Autodesk Inventor part; units mm, degrees
ref_plane "YZ Plane" through (0, 0, 0) normal (1, 0, 0) x (0, 1, 0)
ref_plane "XZ Plane" through (0, 0, 0) normal (0, 1, 0) x (-1, 0, 0)
ref_plane "XY Plane" through (0, 0, 0) normal (0, 0, 1) x (1, 0, 0)
sketch "Sketch1" plane through (0, 0, 0) normal (0, 1, 0) x (-1, 0, 0)
  line L0 (51, -51) -> (-51, -51)
  line L1 (-51, -51) -> (-51, 51)
  line L2 (-51, 51) -> (51, 51)
  line L3 (51, 51) -> (51, -51)
  line L4 (51, -51) -> (-51, 51) construction
  line L5 (-51, -51) -> (51, 51) construction
  point P0 (0, 0)
  dimension "d0" = 102
  dimension "d1" = 102
extrude "Extrusion1" add sketch "Sketch1" along normal blind 17
chamfer "Chamfer1" distance 15 angle 45 4 edges at (51, 8.5, 51) (51, 8.5, -51) (-51, 8.5, -51) (-51, 8.5, 51)
sketch "Sketch2" plane through (0, 17, 0) normal (0, 1, 0) x (1, 0, 0)
  line L0 (51, -36) -> (51, 36)
  line L1 (-51, 36) -> (-51, -36)
  line L2 (51, -36) -> (36, -51)
  line L3 (36, 51) -> (-36, 51)
  circle A0 centre (36, -36) radius 6.5
  circle A1 centre (-36, -36) radius 6.5
  circle A2 centre (36, 36) radius 6.5
  circle A3 centre (-36, 36) radius 6.5
  circle A4 centre (0, 0) radius 23
  dimension "d7" = 13
  dimension "d8" = 13
  dimension "d9" = 13
  dimension "d10" = 13
  dimension "d22" = 46
extrude "Extrusion2" cut sketch "Sketch2" against normal through all contours A0 | A1 | A2 | A3
thread "Thread1"
thread "Thread2"
thread "Thread3"
thread "Thread4"
sketch "Sketch3" plane through (0, 17, 0) normal (0, 1, 0) x (1, 0, 0)
  circle A0 centre (0, 0) radius 23
  dimension "d23" = 46
extrude "Extrusion3" cut sketch "Sketch3" against normal through all
properties part number "00.32.004 \"Flange\"" material "Steel"
Read the model definition and answer for the solid it produces. Units are mm, in the model's axes. Coordinates: 2 decimals unless noted, no trailing zeros. Loops run counter-clockwise (first coordinate to the right, second up) from the corner with the lowest first, then second, coordinate; pieces in that order, holes last.
(1) The part is cut by section B-B (y = 5.75). Determine the outline of the cut face in (x, z), and give its area (3 significant figures).
Solution:
outline: (-51, -36) - (-36, -51) - (36, -51) - (51, -36) - (51, 36) - (36, 51) - (-36, 51) - (-51, 36) - close; hole circle Ø13 at (-36, -36); hole circle Ø13 at (-36, 36); hole circle Ø46 at (0, 0); hole circle Ø13 at (36, -36); hole circle Ø13 at (36, 36)
area: 7,760 mm2
(2) The part is cut by section C-C (x = 0). Determine the outline of the cut face in (y, z), and give its area (3 significant figures).
Solution:
outline: (0, -51) - (17, -51) - (17, -23) - (0, -23) - close; (0, 23) - (17, 23) - (17, 51) - (0, 51) - close
area: 952 mm2
(3) Consider line 1 along X through (y, z) = (13.25, 36); line 2 along Z through (x, y) = (-0.5, 1.5). Determine where each line is inside the solid, lowest interval first.
Solution:
line 1: x = -51 to -42.5, -29.5 to 29.5, 42.5 to 51
line 2: z = -51 to -22.99, 22.99 to 51
(4) The mould has two halves that part along X. Classify faces 1 (the face through (-2.994, 8.619, -22.804)), 2 (the face through (43, 8, 44)), 3 (the face through (0.7, 0, 23.4)): released by +X, released by -X, zero draft, split by the parting line, or undercut.
Solution:
face 1: undercut
face 2: released by +X
face 3: zero draft
(5) The part is cut by section A-A (z = 0). Determine the outline of the cut face in (x, y), and give its area (3 significant figures).
Solution:
outline: (-51, 0) - (-23, 0) - (-23, 17) - (-51, 17) - close; (23, 0) - (51, 0) - (51, 17) - (23, 17) - close
area: 952 mm2
(6) The part is cut by section D-D (z = 37.5). Determine the outline of the cut face in (x, y).
Solution:
outline: (-49.5, 0) - (-42.32, 0) - (-42.32, 17) - (-49.5, 17) - close; (-29.68, 0) - (29.68, 0) - (29.68, 17) - (-29.68, 17) - close; (42.32, 0) - (49.5, 0) - (49.5, 17) - (42.32, 17) - close
(7) Flat-ended cylindrical pins translate along their axes: pin 1 Ø11.5 at (x, z) = (36, 36) entering from +Y; pin 2 Ø1.5 at (x, y) = (-38.5, 14.5) entering from -Z; pin 3 Ø6 at (y, z) = (6, -39.5) entering from +X. Find the tip coordinate at first contact, or state that the pin passes through.
Solution:
pin 1: passes through
pin 2: stops at z = -49.25
pin 3: stops at x = 50.5
